from build123d import *

# Parameters (mm, degrees)
SKETCH1_W                       = 154
SKETCH1_H                       = 270
BOSS_EXTRUDE1_DEPTH             = 140
BOSS_EXTRUDE1_DRAFT             = -10
SKETCH2_W                       = 154
SKETCH2_H                       = 270
BOSS_EXTRUDE2_DEPTH             = 5
BOSS_EXTRUDE3_REACH             = 237.456
BOSS_EXTRUDE3_DIRECTION_2_REACH = 237.456
SHELL1_T                        = -3
SKETCH5_W                       = 15
SKETCH5_H                       = 55
BOSS_EXTRUDE4_DEPTH             = 5
BOSS_EXTRUDE5_DEPTH             = 5
LPATTERN1_COUNT                 = 4
LPATTERN1_PITCH                 = 16.7215
SKETCH7_W                       = 15
SKETCH7_H                       = 0.1645
CUT_EXTRUDE2_DEPTH              = 234.966061846
MIRROR2_START                   = -27.5
MIRROR2_OUTLINE_W               = 15
MIRROR2_OUTLINE_H               = 5
MIRROR2_DEPTH                   = 55
MIRROR2_START_2                 = -10.943
MIRROR2_2_DEPTH                 = 5
MIRROR2_START_3                 = 5.7785
MIRROR2_3_DEPTH                 = 5
MIRROR2_START_4                 = 22.5
MIRROR2_4_DEPTH                 = 5
MIRROR2_5_DEPTH                 = 4.8355
SKETCH8_W                       = 268
SKETCH8_H                       = 1.5
CUT_EXTRUDE3_DEPTH              = 35
SKETCH9_R                       = 19
CUT_EXTRUDE4_DEPTH              = 35
SKETCH10_W                      = 157.371554598
SKETCH10_H                      = 224
CUT_EXTRUDE5_DEPTH              = 35
BOSS_EXTRUDE6_START             = 20
SKETCH11_R                      = 21
SKETCH11_R_2                    = 19
BOSS_EXTRUDE6_DEPTH             = 20
BOSS_EXTRUDE7_START             = 3
SKETCH12_R                      = 29
SKETCH12_R_2                    = 19
BOSS_EXTRUDE7_DEPTH             = 3
CHAMFER1_SIZE                   = 2
BOSS_EXTRUDE8_START             = 137
BOSS_EXTRUDE8_2_OUTLINE_W       = 203.371554598
BOSS_EXTRUDE8_2_OUTLINE_H       = 12.482701107
BOSS_EXTRUDE8_2_DEPTH           = 3


with BuildPart() as part:
    # Sketch1 → Boss-Extrude1 (with draft: the straight prism first)
    with BuildSketch(Plane(origin=(0, 0, 0), x_dir=(1, 0, 0), z_dir=(0, 1, 0))):
        Rectangle(SKETCH1_W, SKETCH1_H)
    extrude(amount=BOSS_EXTRUDE1_DEPTH)
    # Boss-Extrude1: the draft: its side faces are tilted about the plane it starts from
    boss_extrude1_sides = [part.faces().sort_by_distance(p)[0] for p in [
        (-77, 70, 0),
        (0, 70, 135),
        (77, 70, 0),
        (0, 70, -135),
    ]]
    draft(boss_extrude1_sides, Plane(origin=(0, 0, 0), x_dir=(1, 0, 0), z_dir=(0, 1, 0)), BOSS_EXTRUDE1_DRAFT)

    # Sketch2 → Boss-Extrude2 (add)
    with BuildSketch(Plane.XZ):
        Rectangle(SKETCH2_W, SKETCH2_H)
    extrude(amount=BOSS_EXTRUDE2_DEPTH)

    # Boss-Extrude3: up to this plane
    boss_extrude3_end = Plane(origin=(-77, 0, 135), z_dir=(0, -0.17364817766693072, 0.984807753012208))
    # Sketch4 → Boss-Extrude3 (add, up to the surface)
    with BuildSketch(Plane.XY, mode=Mode.PRIVATE) as boss_extrude3_sk1:
        Polygon((101.685777299, -5), (77, -5), (77, 0), (101.685777299, 140), align=None)
    boss_extrude3_tool1 = split(extrude(boss_extrude3_sk1.sketch, amount=BOSS_EXTRUDE3_REACH, mode=Mode.PRIVATE), bisect_by=boss_extrude3_end, keep=Keep.BOTH, mode=Mode.PRIVATE)
    boss_extrude3 = boss_extrude3_tool1.solids().sort_by_distance((93.182898, 43.388889, 0))[0]
    add(boss_extrude3)

    # Boss-Extrude3 direction 2: up to this plane
    boss_extrude3_direction_2_end = Plane(origin=(-77, 0, -135), z_dir=(0, -0.17364817766693072, -0.984807753012208))
    # Sketch4 → Boss-Extrude3 direction 2 (add, up to the surface)
    with BuildSketch(Plane.XY, mode=Mode.PRIVATE) as boss_extrude3_direction_2_sk1:
        Polygon((101.685777299, -5), (77, -5), (77, 0), (101.685777299, 140), align=None)
    boss_extrude3_direction_2_tool1 = split(extrude(boss_extrude3_direction_2_sk1.sketch, amount=-BOSS_EXTRUDE3_DIRECTION_2_REACH, mode=Mode.PRIVATE), bisect_by=boss_extrude3_direction_2_end, keep=Keep.BOTH, mode=Mode.PRIVATE)
    boss_extrude3_direction_2 = boss_extrude3_direction_2_tool1.solids().sort_by_distance((93.182898, 43.388889, 0))[0]
    add(boss_extrude3_direction_2)
    boss_extrude3 = boss_extrude3 + boss_extrude3_direction_2  # both directions under the feature's name, for the pattern or mirror that repeats it

    # Mirror1: Boss-Extrude3 across plane
    add(boss_extrude3.mirror(Plane(origin=(0, 0, 0), x_dir=(0, 0, 1), z_dir=(1, 0, 0))))

    # Shell1
    shell1_openings = [part.faces().sort_by_distance(p)[0] for p in [
        (0, 140, 0),
    ]]
    offset(amount=SHELL1_T, openings=shell1_openings, kind=Kind.INTERSECTION)

    # Sketch5 → Boss-Extrude4 (add)
    with BuildSketch(Plane(origin=(0, 120, 0), x_dir=(1, 0, 0), z_dir=(0, 1, 0))):
        with Locations((109.185777299, 0)):
            Rectangle(SKETCH5_W, SKETCH5_H)
    extrude(amount=BOSS_EXTRUDE4_DEPTH)

    # Sketch6 → Boss-Extrude5 (add)
    with BuildSketch(Plane.XY.offset(27.5)):
        with BuildLine():
            Line((101.685777299, 120), (101.685777299, 95))
            ThreePointArc((101.685777299, 95), (107.105041487, 108.748441487), (116.685777299, 120))
            Line((116.685777299, 120), (101.685777299, 120))
        make_face()
    boss_extrude5 = extrude(amount=-BOSS_EXTRUDE5_DEPTH)

    # LPattern1: Boss-Extrude5 ×4
    with Locations(*[(0, 0, -i * LPATTERN1_PITCH) for i in range(1, LPATTERN1_COUNT)]):
        add(boss_extrude5)

    # Sketch7 → Cut-Extrude2 (cut, through all)
    with BuildSketch(Plane(origin=(0, 120, 0), x_dir=(1, 0, 0), z_dir=(0, 1, 0))):
        with Locations((109.185777299, 27.58225)):
            Rectangle(SKETCH7_W, SKETCH7_H)
    extrude(amount=-CUT_EXTRUDE2_DEPTH, mode=Mode.SUBTRACT)

    # Mirror2: read off the stored shape, not the designer's step
    # Mirror2 outline → Mirror2 (add)
    with BuildSketch(Plane.XY.offset(MIRROR2_START)):
        with Locations((-109.185777299, 122.5)):
            Rectangle(MIRROR2_OUTLINE_W, MIRROR2_OUTLINE_H)
    extrude(amount=MIRROR2_DEPTH)

    # Mirror2 2 outline → Mirror2 2 (add)
    with BuildSketch(Plane.XY.offset(MIRROR2_START_2)):
        with BuildLine():
            ThreePointArc((-116.685777299, 120), (-107.105041487, 108.748441487), (-101.685777299, 95))
            Line((-101.685777299, 95), (-101.685777299, 120))
            Line((-101.685777299, 120), (-116.685777299, 120))
        make_face()
    extrude(amount=MIRROR2_2_DEPTH)

    # Mirror2 3 outline → Mirror2 3 (add)
    with BuildSketch(Plane.XY.offset(MIRROR2_START_3)):
        with BuildLine():
            ThreePointArc((-116.685777299, 120), (-107.105041487, 108.748441487), (-101.685777299, 95))
            Line((-101.685777299, 95), (-101.685777299, 120))
            Line((-101.685777299, 120), (-116.685777299, 120))
        make_face()
    extrude(amount=MIRROR2_3_DEPTH)

    # Mirror2 4 outline → Mirror2 4 (add)
    with BuildSketch(Plane.XY.offset(MIRROR2_START_4)):
        with BuildLine():
            ThreePointArc((-116.685777299, 120), (-107.105041487, 108.748441487), (-101.685777299, 95))
            Line((-101.685777299, 95), (-101.685777299, 120))
            Line((-101.685777299, 120), (-116.685777299, 120))
        make_face()
    extrude(amount=MIRROR2_4_DEPTH)

    # Mirror2 5 outline → Mirror2 5 (add)
    with BuildSketch(Plane.XY.offset(MIRROR2_START)):
        with BuildLine():
            ThreePointArc((-116.685777299, 120), (-107.105041487, 108.748441487), (-101.685777299, 95))
            Line((-101.685777299, 95), (-101.685777299, 120))
            Line((-101.685777299, 120), (-116.685777299, 120))
        make_face()
    extrude(amount=MIRROR2_5_DEPTH)

    # Sketch8 → Cut-Extrude3 (cut)
    with BuildSketch(Plane(origin=(101.685777299, 0, 0), x_dir=(0, 0, -1), z_dir=(1, 0, 0))):
        with Locations((0, -2.75)):
            Rectangle(SKETCH8_W, SKETCH8_H)
    extrude(amount=-CUT_EXTRUDE3_DEPTH, mode=Mode.SUBTRACT)

    # Sketch9 → Cut-Extrude4 (cut)
    with BuildSketch(Plane.ZY.offset(101.685777299)):
        with Locations(Location((0, 20, 0), (0, 0, 270))):
            Circle(SKETCH9_R)
    extrude(amount=-CUT_EXTRUDE4_DEPTH, mode=Mode.SUBTRACT)

    # Sketch10 → Cut-Extrude5 (cut)
    with BuildSketch(Plane(origin=(0, -2, 0), x_dir=(1, 0, 0), z_dir=(0, 1, 0))):
        Rectangle(SKETCH10_W, SKETCH10_H)
    extrude(amount=-CUT_EXTRUDE5_DEPTH, mode=Mode.SUBTRACT)

    # Sketch11 → Boss-Extrude6 (add)
    with BuildSketch(Plane.ZY.offset(101.685777299).offset(BOSS_EXTRUDE6_START)):
        with Locations(Location((0, 20, 0), (0, 0, 90))):
            Circle(SKETCH11_R)
        with Locations(Location((0, 20, 0), (0, 0, 270))):
            Circle(SKETCH11_R_2, mode=Mode.SUBTRACT)
    extrude(amount=-BOSS_EXTRUDE6_DEPTH)

    # Sketch12 → Boss-Extrude7 (add)
    with BuildSketch(Plane.ZY.offset(121.685777299).offset(BOSS_EXTRUDE7_START)):
        with Locations(Location((0, 20, 0), (0, 0, 270))):
            Circle(SKETCH12_R)
        with Locations(Location((0, 20, 0), (0, 0, 270))):
            Circle(SKETCH12_R_2, mode=Mode.SUBTRACT)
    extrude(amount=-BOSS_EXTRUDE7_DEPTH)

    # Chamfer1
    chamfer1_edges = [part.edges().sort_by_distance(p)[0] for p in [
        (-98.685777299, 39, 0),
    ]]
    chamfer(chamfer1_edges, length=CHAMFER1_SIZE)

    # Boss-Extrude8: read off the stored shape, not the designer's step
    # Boss-Extrude8 outline → Boss-Extrude8 (revolve)
    with BuildSketch(Plane(origin=(0, 20, 0), x_dir=(0, 1, 0), z_dir=(0, 0, -1))):
        Polygon((23, -121.685777299), (21, -119.685777299), (21, -121.685777299), align=None)
        Polygon((21, -101.685777299), (21, -103.685777299), (23, -101.685777299), align=None)
    boss_extrude8 = revolve(axis=Axis((0, 20, 0), (1, 0, 0)))

    # Boss-Extrude8 2 outline → Boss-Extrude8 2 (add)
    with BuildSketch(Plane(origin=(0, 0, 0), x_dir=(1, 0, 0), z_dir=(0, 1, 0)).offset(BOSS_EXTRUDE8_START)):
        with Locations((0, -165.398146911)):
            Rectangle(BOSS_EXTRUDE8_2_OUTLINE_W, BOSS_EXTRUDE8_2_OUTLINE_H)
    boss_extrude8_2 = extrude(amount=BOSS_EXTRUDE8_2_DEPTH)

    # Mirror3: Boss-Extrude8, Boss-Extrude8 2 across plane
    add(boss_extrude8.mirror(Plane.XY))
    add(boss_extrude8_2.mirror(Plane.XY))


solid = part.part
Input: part model. Units: mm. Frame: model coordinates. A direction names the side the tool comes from. Round coordinates to 2 decimals unless told otherwise and drop trailing zeros. Order: outer loops, then holes, each group sorted by start corner. A loop starts at its lowest first (then second) coordinate and runs counter-clockwise, first axis right, second up.
1. Cut plane D-D, the plane z = 0. State how many separate pieces and enclosed holes the cut face has, then the cut area to 3 significant figures.
The answers:
separate pieces: 4
enclosed holes: 0
area: 1,140 mm2
2. Cut plane C-C, the plane y = 91. Output: boundary loops of the cut face in (x, z), then the cut area to 3 significant figures.
The answers:
outline: (-101.69, -151.05) - (101.69, -151.05) - (101.69, 151.05) - (-101.69, 151.05) - close; hole (-98.69, -148) - (98.69, -148) - (98.69, 148) - (-98.69, 148) - close
area: 3,020 mm2
3. Cut plane B-B, the plane z = -56.5. Output: boundary loops of the cut face in (x, y).
The answers:
outline: (-101.69, -5) - (-78.69, -5) - (-78.69, -2) - (-98.69, -2) - (-98.69, 140) - (-101.69, 140) - close; (78.69, -5) - (101.69, -5) - (101.69, -3.5) - (78.69, -3.5) - close; (98.69, -2) - (101.69, -2) - (101.69, 140) - (98.69, 140) - close
4. Material intervals for line 1 (X direction, y = 81, z = -25); line 2 (Z direction, x = -119, y = 20); line 3 (Z direction, x = 77, y = 14), sorted ascending.
The answers:
line 1: x = -101.69 to -98.69, 98.69 to 101.69
line 2: z = -21 to -19, 19 to 21
line 3: z = -137.47 to -134.42, 134.42 to 137.47
5. Mould query, pull axis Z, two halves, no side actions, for faces 4 (the face through (0, 140, 166)), 5 (the face through (106, 113, 22.5)), 6 (the face through (-111.8, 4.52, -14.19)), 7 (the face through (107, 117, 27.5)). Classes: released by +Z, released by -Z, zero draft, split by the parting line, or undercut.
The answers:
face 4: zero draft
face 5: undercut
face 6: split by the parting line
face 7: released by +Z
6. Set-up query: faces 1 (the face through (-108, 117, 27.5)), 2 (the face through (-109, 120, -17)), 3 (the face through (107, 117, -27.5)). Return all of +Z, -Z, +X, -X, +Y, -Y with unobstructed straight access to the full face (end or side cutting, diameter ignored); none if empty.
The answers:
face 1: +Z, -X, +Y, -Y
face 2: -X
face 3: -Z, +X, +Y, -Y
7. Pin query (flat end, axial travel): P1, Ø13, axis at x = -112.5, z = -2.5, coming from the -Y side; P2, Ø10, axis at x = -69.5, y = 114, coming from the -Z side; P3, Ø0.8, axis at y = -3, z = -122.5, coming from the +X side. Return the tip coordinate at first contact, or that it passes through.
The answers:
P1: stops at y = -1
P2: stops at z = -155.98
P3: stops at x = 66.69
8. Cut plane A-A, the plane x = 3. Output: boundary loops of the cut face in (y, z).
The answers:
outline: (-5, -135) - (0, -135) - (137, -159.16) - (137, -171.64) - (140, -171.64) - (140, -156.64) - (0.26, -132) - (-2, -132) - (-2, -112) - (-5, -112) - close; (-5, 112) - (-2, 112) - (-2, 132) - (0.26, 132) - (140, 156.64) - (140, 171.64) - (137, 171.64) - (137, 159.16) - (0, 135) - (-5, 135) - close
